from build123d import *

# Parameters (mm, degrees)
F0_W     = 9.525
F0_H     = 9.271
F1_DEPTH = 31.75
F2_R     = 4.0386
F3_DEPTH = 5.08
F4_R     = 2.2225
F5_DEPTH = 4.192


with BuildPart() as f1:
    # F0 (on Front) → F1 (new body)
    with BuildSketch(Plane.XZ):
        with Locations((4.7625, 4.6355)):
            Rectangle(F0_W, F0_H)
    extrude(amount=F1_DEPTH)

    # F2 (on face) → F3 (cut)
    with BuildSketch(Plane.XY.offset(9.271)):
        with Locations((4.7625, -15.875)):
            Circle(F2_R)
    extrude(amount=-F3_DEPTH, mode=Mode.SUBTRACT)

    # F4 (on face) → F5 (cut, through all)
    with BuildSketch(Plane.XY.offset(4.191)):
        with Locations((4.7625, -15.875)):
            Circle(F4_R)
    extrude(amount=-F5_DEPTH, mode=Mode.SUBTRACT)


solid = f1.part
The listing builds one solid part. Answer for the finished solid, in the listing's coordinates (mm). A direction names the side the tool comes from. Give positions to 0.01 mm unless a question says otherwise; leave off trailing zeros. Order: outer loops, then holes, each group sorted by start corner. A loop starts at its lowest first (then second) coordinate and runs counter-clockwise, first axis right, second up. Notation, with made-up numbers: (44.5, 44.5) - (74.5, 44.5) arc R25 ccw to (74.5, 76.5) - close; hole circle Ø6 at (45.25, 34). An arc over 180 degrees is marked (long way). One line per item, written item: value. Start each with the question number.
1) Given pin 1 Ø4 at (x, y) = (2, -26.5) entering from -Z, flat-ended and moving along its own axis, determine where the tip first touches the part or whether it passes through.
2) A tool of negligible diameter and unlimited length cuts with its end or side. For faces 1 (the face through (7, -12, 9.271)), 2 (the face through (7, -18, 4.191)), from which of +Z, -Z, +X, -X, +Y, -Y can it reach the whole face along a straight path? Write none if from no direction.
3) A cutting plane is placed at B-B on y = -17. Give the vertices of the cut face in (x, z) (3 decimals).
4) A cutting plane is placed at D-D on x = 8. Give the vertices of the cut face in (y, z), then the cut area to 3 significant figures.
5) The mould has two halves that part along Y. Classify faces 3 (the face through (5, 0, 5)), 4 (the face through (9.525, -16, 5)), 5 (the face through (1.558, -18.332, 6.767)): released by +Y, released by -Y, zero draft, split by the parting line, or undercut.
6) A cutting plane is placed at A-A on x = 3.25. Give the vertices of the cut face in (y, z).
7) Find the intervals of material crossed by L1, parallel to X at y = -12.5, z = 7.25 (3 decimals); L2, parallel to Y at x = 6, z = 1.5; L3, parallel to Y at x = 4.25, z = 8.5, in increasing order.
Answer sheet:
1. pin 1: stops at z = 0
2. face 1: +Z, +X, -X, +Y, -Y
2. face 2: +Z
3. outline: (0, 0) - (2.846, 0) - (2.846, 4.191) - (0.884, 4.191) - (0.884, 9.271) - (0, 9.271) - close; (6.679, 0) - (9.525, 0) - (9.525, 9.271) - (8.641, 9.271) - (8.641, 4.191) - (6.679, 4.191) - close
4. outline: (-31.75, 0) - (0, 0) - (0, 9.27) - (-13.46, 9.27) - (-13.46, 4.19) - (-18.29, 4.19) - (-18.29, 9.27) - (-31.75, 9.27) - close
4. area: 270 mm2
5. face 3: released by +Y
5. face 4: zero draft
5. face 5: undercut
6. outline: (-31.75, 0) - (-17.5, 0) - (-17.5, 4.19) - (-19.62, 4.19) - (-19.62, 9.27) - (-31.75, 9.27) - close; (-14.25, 0) - (0, 0) - (0, 9.27) - (-12.13, 9.27) - (-12.13, 4.19) - (-14.25, 4.19) - close
7. L1: x = 0 to 2.544, 6.981 to 9.525
7. L2: y = -31.75 to -17.72, -14.03 to 0
7. L3: y = -31.75 to -19.88, -11.87 to 0
